Read the model definition and answer for the solid it produces. Units are mm, in the model's axes. A direction names the side the tool comes from. Give positions to 0.01 mm unless a question says otherwise; leave off trailing zeros. Order: outer loops, then holes, each group sorted by start corner. A loop starts at its lowest first (then second) coordinate and runs counter-clockwise, first axis right, second up. Notation, with made-up numbers: (41, 56.5) -> (76, 56.5) arc R13 cw to (76, 62.5) -> close; hole circle Ø1 at (4.25, -33.5). An arc over 180 degrees is marked (long way). One line per item, written item: value. Start each with the question number.
from build123d import *
from OCP.BRepFilletAPI import BRepFilletAPI_MakeChamfer

# Parameters (mm, degrees)
BOSS_EXTRUDE1_DEPTH                            = 6.35
FILLET5_R                                      = 19.05
FILLET6_R                                      = 19.05
FILLET7_R                                      = 19.05
FILLET8_R                                      = 19.05
CUT_EXTRUDE1_DEPTH                             = 532.923850283
CUT_EXTRUDE2_DEPTH                             = 532.923850283
CHAMFER1_SIZE                                  = 4.0894
CHAMFER1_SIZE2                                 = 3.682112299
CHAMFER2_SIZE                                  = 4.0894
CHAMFER2_SIZE2                                 = 3.682112299
F_62_0_038_DIAMETER_HOLE1_D                    = 0.9652
F_62_0_038_DIAMETER_HOLE1_DEPTH                = 25.4
F_62_0_038_DIAMETER_HOLE1_TIP                  = 0.289975335
CSK_FOR_4_FLAT_HEAD_MACHINE_SCREW3_D           = 3.2639
CSK_FOR_4_FLAT_HEAD_MACHINE_SCREW3_CSINK_D     = 5.715
CSK_FOR_4_FLAT_HEAD_MACHINE_SCREW3_CSINK_ANGLE = 82


with BuildPart() as part:
    # Sketch1 → Boss-Extrude1 (new body)
    with BuildSketch(Plane.XY):
        Polygon((0, 0), (0, -292.1), (444.5, -292.1), (444.5, 0), (393.7, 0), (393.7, -241.3), (50.8, -241.3), (50.8, 0), align=None)
    extrude(amount=BOSS_EXTRUDE1_DEPTH)

    # Fillet5
    fillet5_edges = [part.edges().sort_by_distance(p)[0] for p in [
        (0, -292.1, 3.175),
    ]]
    fillet(fillet5_edges, radius=FILLET5_R)

    # Fillet6
    fillet6_edges = [part.edges().sort_by_distance(p)[0] for p in [
        (444.5, -292.1, 3.175),
    ]]
    fillet(fillet6_edges, radius=FILLET6_R)

    # Fillet7
    fillet7_edges = [part.edges().sort_by_distance(p)[0] for p in [
        (50.8, -241.3, 3.175),
    ]]
    fillet(fillet7_edges, radius=FILLET7_R)

    # Fillet8
    fillet8_edges = [part.edges().sort_by_distance(p)[0] for p in [
        (393.7, -241.3, 3.175),
    ]]
    fillet(fillet8_edges, radius=FILLET8_R)

    # Sketch2 → Cut-Extrude1 (cut, through all)
    with BuildSketch(Plane.XY.offset(6.35)):
        with BuildLine():
            Line((422.3639, -107.95), (422.3639, -260.35))
            ThreePointArc((422.3639, -260.35), (419.1, -263.6139), (415.8361, -260.35))
            Line((415.8361, -260.35), (415.8361, -107.95))
            ThreePointArc((415.8361, -107.95), (419.1, -104.6861), (422.3639, -107.95))
        make_face()
    extrude(amount=-CUT_EXTRUDE1_DEPTH, mode=Mode.SUBTRACT)

    # Sketch3 → Cut-Extrude2 (cut, through all)
    with BuildSketch(Plane.XY.offset(6.35)):
        with BuildLine():
            Line((28.6639, -107.95), (28.6639, -260.35))
            ThreePointArc((28.6639, -260.35), (25.4, -263.6139), (22.1361, -260.35))
            Line((22.1361, -260.35), (22.1361, -107.95))
            ThreePointArc((22.1361, -107.95), (25.4, -104.6861), (28.6639, -107.95))
        make_face()
    extrude(amount=-CUT_EXTRUDE2_DEPTH, mode=Mode.SUBTRACT)

    # Sketch4 → CSK for 1/4 Flat Head Machine Screw1 (revolve, cut)
    with BuildSketch(Plane(origin=(425.45, -50.8, 0), x_dir=(0, 1, 0), z_dir=(1, 0, 0))):
        Polygon((0, 0), (0, 6.35), (3.3782, 6.35), (3.3782, 3.520932584), (6.4389, 0), align=None)
    revolve(axis=Axis((425.45, -50.8, -6.35), (0, 0, 1)), mode=Mode.SUBTRACT)

    # Chamfer1: one chamfer whose edges measure the first distance from different faces: ONE call of the kernel's chamfer builder (chamfer() names one face for all edges)
    chamfer1_edges_1 = [part.edges().sort_by_distance(p)[0] for p in [
        (25.4, -104.6861, 0),
    ]]
    chamfer1_side_1 = [part.faces().sort_by_distance(p)[0] for p in [
        (25.4, -104.6861, 3.175),
    ]]
    chamfer1_edges_2 = [part.edges().sort_by_distance(p)[0] for p in [
        (28.6639, -184.15, 0),
    ]]
    chamfer1_side_2 = [part.faces().sort_by_distance(p)[0] for p in [
        (28.6639, -184.15, 3.175),
    ]]
    chamfer1_edges_3 = [part.edges().sort_by_distance(p)[0] for p in [
        (25.4, -263.6139, 0),
    ]]
    chamfer1_side_3 = [part.faces().sort_by_distance(p)[0] for p in [
        (25.4, -263.6139, 3.175),
    ]]
    chamfer1_edges_4 = [part.edges().sort_by_distance(p)[0] for p in [
        (22.1361, -184.15, 0),
    ]]
    chamfer1_side_4 = [part.faces().sort_by_distance(p)[0] for p in [
        (22.1361, -184.15, 3.175),
    ]]
    chamfer1 = BRepFilletAPI_MakeChamfer(part.part.solid().wrapped)
    for e in chamfer1_edges_1:
        chamfer1.Add(CHAMFER1_SIZE, CHAMFER1_SIZE2, e.wrapped, chamfer1_side_1[0].wrapped)  # the first distance lies on this face
    for e in chamfer1_edges_2:
        chamfer1.Add(CHAMFER1_SIZE, CHAMFER1_SIZE2, e.wrapped, chamfer1_side_2[0].wrapped)  # the first distance lies on this face
    for e in chamfer1_edges_3:
        chamfer1.Add(CHAMFER1_SIZE, CHAMFER1_SIZE2, e.wrapped, chamfer1_side_3[0].wrapped)  # the first distance lies on this face
    for e in chamfer1_edges_4:
        chamfer1.Add(CHAMFER1_SIZE, CHAMFER1_SIZE2, e.wrapped, chamfer1_side_4[0].wrapped)  # the first distance lies on this face
    add(Compound.cast(chamfer1.Shape()), mode=Mode.REPLACE)

    # Chamfer2: one chamfer whose edges measure the first distance from different faces: ONE call of the kernel's chamfer builder (chamfer() names one face for all edges)
    chamfer2_edges_1 = [part.edges().sort_by_distance(p)[0] for p in [
        (419.1, -104.6861, 0),
    ]]
    chamfer2_side_1 = [part.faces().sort_by_distance(p)[0] for p in [
        (419.1, -104.6861, 3.175),
    ]]
    chamfer2_edges_2 = [part.edges().sort_by_distance(p)[0] for p in [
        (422.3639, -184.15, 0),
    ]]
    chamfer2_side_2 = [part.faces().sort_by_distance(p)[0] for p in [
        (422.3639, -184.15, 3.175),
    ]]
    chamfer2_edges_3 = [part.edges().sort_by_distance(p)[0] for p in [
        (419.1, -263.6139, 0),
    ]]
    chamfer2_side_3 = [part.faces().sort_by_distance(p)[0] for p in [
        (419.1, -263.6139, 3.175),
    ]]
    chamfer2_edges_4 = [part.edges().sort_by_distance(p)[0] for p in [
        (415.8361, -184.15, 0),
    ]]
    chamfer2_side_4 = [part.faces().sort_by_distance(p)[0] for p in [
        (415.8361, -184.15, 3.175),
    ]]
    chamfer2 = BRepFilletAPI_MakeChamfer(part.part.solid().wrapped)
    for e in chamfer2_edges_1:
        chamfer2.Add(CHAMFER2_SIZE, CHAMFER2_SIZE2, e.wrapped, chamfer2_side_1[0].wrapped)  # the first distance lies on this face
    for e in chamfer2_edges_2:
        chamfer2.Add(CHAMFER2_SIZE, CHAMFER2_SIZE2, e.wrapped, chamfer2_side_2[0].wrapped)  # the first distance lies on this face
    for e in chamfer2_edges_3:
        chamfer2.Add(CHAMFER2_SIZE, CHAMFER2_SIZE2, e.wrapped, chamfer2_side_3[0].wrapped)  # the first distance lies on this face
    for e in chamfer2_edges_4:
        chamfer2.Add(CHAMFER2_SIZE, CHAMFER2_SIZE2, e.wrapped, chamfer2_side_4[0].wrapped)  # the first distance lies on this face
    add(Compound.cast(chamfer2.Shape()), mode=Mode.REPLACE)

    # #62 (0.038) Diameter Hole1
    with Locations(Plane.XY.offset(6.35)):
        with Locations((42.8625, -73.025), (42.8625, -79.375)):
            Hole(F_62_0_038_DIAMETER_HOLE1_D / 2, depth=F_62_0_038_DIAMETER_HOLE1_DEPTH)
            with Locations((0, 0, -(F_62_0_038_DIAMETER_HOLE1_DEPTH + F_62_0_038_DIAMETER_HOLE1_TIP / 2))):  # 118° drill point
                Cone(0, F_62_0_038_DIAMETER_HOLE1_D / 2, F_62_0_038_DIAMETER_HOLE1_TIP, mode=Mode.SUBTRACT)

    # CSK for #4 Flat Head Machine Screw3 (through all)
    with Locations(Plane(origin=(0, 0, 0), x_dir=(-1, 0, 0), z_dir=(0, 0, -1))):
        with Locations((-42.8625, -79.375), (-42.8625, -73.025)):
            CounterSinkHole(CSK_FOR_4_FLAT_HEAD_MACHINE_SCREW3_D / 2, CSK_FOR_4_FLAT_HEAD_MACHINE_SCREW3_CSINK_D / 2, counter_sink_angle=CSK_FOR_4_FLAT_HEAD_MACHINE_SCREW3_CSINK_ANGLE)


solid = part.part
Item 1: Find the intervals of material crossed by line 1 (X direction, y = -259, z = 6); line 2 (Y direction, x = 425.45, z = 4.85); line 3 (X direction, y = -40, z = 2), in increasing order. Write a range as from..to.
Item 2: Flat-ended cylindrical pins translate along their axes: pin 1 (2.5 mm diameter, centred on x = 42.86, y = -73.03, fed in from +Z); pin 2 (1 mm diameter, centred on x = 92.5, z = 4.5, fed in from +Y). Find the tip coordinate at first contact, or state that the pin passes through.
Item 3: Find section C-C on x = 315. Write down the section's boundary in (y, z).
Item 4: A tool of negligible diameter and unlimited length cuts with its end or side. For faces 1 (the cylindrical face through (5.43, -286.37, 3.22)), 2 (the cylindrical face through (56.23, -235.57, 3.22)), from which of +Z, -Z, +X, -X, +Y, -Y can it reach the whole face along a straight path? Write none if from no direction.
Item 5: Find section D-D on x = 64. Write down the section's boundary in (y, z), then the cut area to 3 significant figures.
Item 6: Find section A-A on y = -130.5. Write down the section's boundary in (x, z), then the cut area to 3 significant figures.
Item 7: Find section B-B on y = -64. Write down the section's boundary in (x, z).
Item 8: For a pull along Y with two mould halves and no side action, classify faces 3 (the conical face through (428.935, -51.574, 3.301)), 4 (the cylindrical face through (387.97, -235.87, 3.22)), 5 (the cylindrical face through (438.77, -286.67, 3.22)) as +Y half, -Y half, draft (parallel to the pull), parting line (faces both ways), or undercut.
Checks:
1. line 1: 0..22.14, 28.66..415.84, 422.36..444.5
1. line 2: -292.1..-54.18, -47.42..0
1. line 3: 0..50.8, 393.7..444.5
2. pin 1: through
2. pin 2: y = -241.3
3. outline: (-292.1, 0) -> (-241.3, 0) -> (-241.3, 6.35) -> (-292.1, 6.35) -> close
4. face 1: +Z, -Z, -X, -Y
4. face 2: +Z, -Z, +Y
5. outline: (-292.1, 0) -> (-240.38, 0) -> (-240.38, 6.35) -> (-292.1, 6.35) -> close
5. area: 328 mm2
6. outline: (0, 0) -> (18.45, 0) -> (22.14, 4.09) -> (22.14, 6.35) -> (0, 6.35) -> close; (28.66, 4.09) -> (32.35, 0) -> (50.8, 0) -> (50.8, 6.35) -> (28.66, 6.35) -> close; (393.7, 0) -> (412.15, 0) -> (415.84, 4.09) -> (415.84, 6.35) -> (393.7, 6.35) -> close; (422.36, 4.09) -> (426.05, 0) -> (444.5, 0) -> (444.5, 6.35) -> (422.36, 6.35) -> close
6. area: 532 mm2
7. outline: (0, 0) -> (50.8, 0) -> (50.8, 6.35) -> (0, 6.35) -> close; (393.7, 0) -> (444.5, 0) -> (444.5, 6.35) -> (393.7, 6.35) -> close
8. face 3: undercut
8. face 4: +Y half
8. face 5: -Y half
